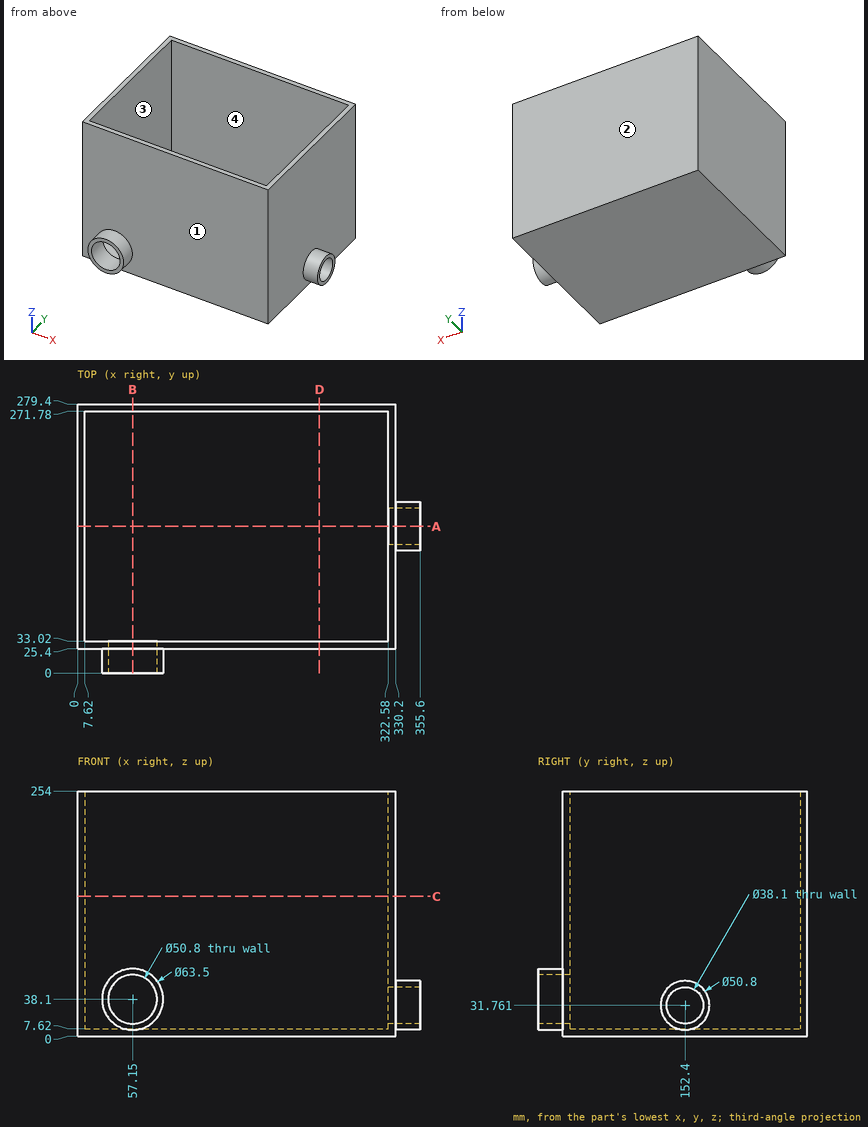
The figure shows three views and two pictorial views of one solid part (mm, origin at its lowest corner). Answer the questions. Give positions to 0.01 mm unless a question says otherwise; leave off trailing zeros. Order: outer loops, then holes, each group sorted by start corner. A loop starts at its lowest first (then second) coordinate and runs counter-clockwise, first axis right, second up. Notation, with made-up numbers: (30, -16.5) -> (76, -16.5) arc R21 cw to (76, 21.5) -> close; hole circle Ø2 at (44.5, -37.5). An arc over 180 degrees is marked (long way). Write each question's results on one line, items separated by ' | '.
Q1. The part is cut by section B-B, the plane x = 57.15. Give the vertices of the cut face in (y, z).
Checked values:
outline: (0, 6.35) -> (25.4, 6.35) -> (25.4, 0) -> (279.4, 0) -> (279.4, 254) -> (271.78, 254) -> (271.78, 7.62) -> (33.02, 7.62) -> (33.02, 12.7) -> (0, 12.7) -> close; (0, 63.5) -> (33.02, 63.5) -> (33.02, 254) -> (25.4, 254) -> (25.4, 69.85) -> (0, 69.85) -> close
Q2. The part is cut by section D-D, the plane x = 251. Give the vertices of the cut face in (y, z).
Checked values:
outline: (25.4, 0) -> (279.4, 0) -> (279.4, 254) -> (271.78, 254) -> (271.78, 7.62) -> (33.02, 7.62) -> (33.02, 254) -> (25.4, 254) -> close
Q3. Straight lines are drawn through the part: probe 1 along Y at (x, z) = (181.5, 86.5); probe 2 along X at (y, z) = (209.5, 208); probe 3 along Z at (x, y) = (57, 26). For each, find the intervals that lie inside material, in ascending order. Write a range as from..to.
Checked values:
probe 1: y = 25.4..33.02, 271.78..279.4 | probe 2: x = 0..7.62, 322.58..330.2 | probe 3: z = 0..12.7, 63.5..254
Q4. Determine the mould class of the marked faces 1, 2, 3 and 4 for opening direction Y: pulls with the +Y half, pulls with the -Y half, needs draft (parallel to the pull), parting line crosses it, or undercut.
Checked values:
face 1: pulls with the -Y half | face 2: pulls with the +Y half | face 3: undercut | face 4: undercut
Q5. Each of these flat-tipped pins is pushed along its axis until it touches: P1, Ø8, axis at y = 207.5, z = 128.5, coming from the +X side; P2, Ø8, axis at x = 45, z = 201.5, coming from the -Y side. Where does it stop, or does it pass through?
Checked values:
P1: stops at x = 330.2 | P2: stops at y = 25.4
Q6. The part is cut by section C-C, the plane z = 145. Give the vertices of the cut face in (x, y).
Checked values:
outline: (0, 25.4) -> (330.2, 25.4) -> (330.2, 279.4) -> (0, 279.4) -> close; hole (7.62, 33.02) -> (322.58, 33.02) -> (322.58, 271.78) -> (7.62, 271.78) -> close
Q7. The part is cut by section A-A, the plane y = 152.4. Give the vertices of the cut face in (x, z), and give its area (3 significant figures).
Checked values:
outline: (0, 0) -> (330.2, 0) -> (330.2, 6.36) -> (355.6, 6.36) -> (355.6, 12.71) -> (322.58, 12.71) -> (322.58, 7.62) -> (7.62, 7.62) -> (7.62, 254) -> (0, 254) -> close; (322.58, 50.81) -> (355.6, 50.81) -> (355.6, 57.16) -> (330.2, 57.16) -> (330.2, 254) -> (322.58, 254) -> close | area: 6,300 mm^2
